Work out the finished part from the listing and answer in its coordinate system (mm). A direction names the side the tool comes from. Round coordinates to 2 decimals unless told otherwise and drop trailing zeros. Write each loop counter-clockwise with the first axis right and the second up, starting at its lowest first coordinate (ties: lowest second). Pieces come first, ordered by that corner, then holes. Notation, with made-up numbers: M 45.5,45 L 103.5,45 A14 cw 103.5,58 Z; hole C -32.5,72.5 d2. An arc over 180 degrees is marked long. One line per item, written item: value. Start each with the question number.
Q1. Find section B-B (x = -47.5). Write down the section's boundary in (y, z).
Q2. Find section A-A (y = -36). Write down the section's boundary in (x, z), and give its area (3 significant figures).
Q3. Given pin 1 Ø9.5 at (x, z) = (-54, 14.5) entering from +Y; pin 2 Ø6 at (y, z) = (-36.5, 6) entering from -X; pin 3 Ø5 at (x, z) = (59.5, 10.5) entering from +Y; pin 4 Ø4 at (x, y) = (-71, -22.5) entering from -Z, each flat-ended and moving along its own axis, determine where each tip first touches the part or whether it passes through.
Q4. Find section C-C (y = -12). Write down the section's boundary in (x, z).
Q5. A tool of negligible diameter and unlimited length cuts with its end or side. For faces 4 (the cylindrical face through (-20.524, -42.135, 10.367)), 5 (the flat face through (64.972, -31, 10)), 6 (the flat face through (78, 26.791, 12)), from which of +Z, -Z, +X, -X, +Y, -Y can it reach the whole face along a straight path? Write none if from no direction.
Q6. Consider probe 1 along X at (y, z) = (30.7, 10); probe 2 along X at (y, z) = (-19.5, 16.75); probe 3 along X at (y, z) = (-50, 12.75). Determine where each line is inside the solid, lowest interval first.
Q7. The mould has two halves that part along Z. Classify faces 1 (the flat face through (-5, -44, 20)), 2 (the conical face through (79.876, 29.058, 10.66)), 3 (the flat face through (-4, -40.709, 10)): released by +Z, released by -Z, zero draft, split by the parting line, or undercut.
from build123d import *

# Parameters (mm, degrees)
F1_DEPTH             = 20
F4_D                 = 4.2
F4_CSINK_D           = 8.2
F4_CSINK_ANGLE       = 80
F4_ON_F2_D           = 4.2
F4_ON_F2_CSINK_D     = 8.2
F4_ON_F2_CSINK_ANGLE = 80
F5_T1_DEPTH          = 20
F5_T3_DEPTH          = 25
F6_R                 = 5
F7_R                 = 1


# Not quite as in the source:
# - a fillet or chamfer that OpenCascade refuses, or shapes differently, is made with other operations: its cross-section is extruded or revolved along the edge and cut away or added


with BuildPart() as f1:
    # F0 (on Top) → F1 (new body)
    with BuildSketch(Plane.XY):
        with BuildLine():
            Line((-74.0278660059, -17.2093475759), (-70.5278660059, -17.2093475759))
            Line((-70.5278660059, -17.2093475759), (-70.5278660059, -4.2093475759))
            Line((-70.5278660059, -4.2093475759), (-74.0278660059, -4.2093475759))
            Line((-74.0278660059, -4.2093475759), (-74.0278660059, 33.7906524241))
            Line((-74.0278660059, 33.7906524241), (-81.0278660059, 33.7906524241))
            Line((-81.0278660059, 33.7906524241), (-96.0278660059, 33.7906524241))
            Line((-96.0278660059, 33.7906524241), (-96.0278660059, 26.7906524241))
            Line((-96.0278660059, 26.7906524241), (-86.0278660059, 26.7906524241))
            ThreePointArc((-86.0278660059, 26.7906524241), (-82.4923321, 25.32618633), (-81.0278660059, 21.7906524241))
            Line((-81.0278660059, 21.7906524241), (-81.0278660059, -48.7093475759))
            Line((-81.0278660059, -48.7093475759), (-81.0278660059, -50.7093475759))
            ThreePointArc((-81.0278660059, -50.7093475759), (-79.5633999118, -54.2448814818), (-76.0278660059, -55.7093475759))
            Line((-76.0278660059, -55.7093475759), (-48.0278660059, -55.7093475759))
            Line((-48.0278660059, -55.7093475759), (-4.5278660059, -55.7093475759))
            Line((-4.5278660059, -55.7093475759), (38.9721339941, -55.7093475759))
            Line((38.9721339941, -55.7093475759), (66.9721339941, -55.7093475759))
            ThreePointArc((66.9721339941, -55.7093475759), (70.5076679, -54.2448814818), (71.9721339941, -50.7093475759))
            Line((71.9721339941, -50.7093475759), (71.9721339941, -48.7093475759))
            Line((71.9721339941, -48.7093475759), (71.9721339941, 21.7906524241))
            ThreePointArc((71.9721339941, 21.7906524241), (73.4366000882, 25.32618633), (76.9721339941, 26.7906524241))
            Line((76.9721339941, 26.7906524241), (86.9721339941, 26.7906524241))
            Line((86.9721339941, 26.7906524241), (86.9721339941, 33.7906524241))
            Line((86.9721339941, 33.7906524241), (71.9721339941, 33.7906524241))
            Line((71.9721339941, 33.7906524241), (64.9721339941, 33.7906524241))
            Line((64.9721339941, 33.7906524241), (64.9721339941, -4.2093475759))
            Line((64.9721339941, -4.2093475759), (61.4721339941, -4.2093475759))
            Line((61.4721339941, -4.2093475759), (61.4721339941, -17.2093475759))
            Line((61.4721339941, -17.2093475759), (64.9721339941, -17.2093475759))
            Line((64.9721339941, -17.2093475759), (64.9721339941, -48.7093475759))
            Line((64.9721339941, -48.7093475759), (12.9721339941, -48.7093475759))
            Line((12.9721339941, -48.7093475759), (12.9721339941, -45.7093475759))
            ThreePointArc((12.9721339941, -45.7093475759), (11.5076679, -42.17381367), (7.9721339941, -40.7093475759))
            Line((7.9721339941, -40.7093475759), (-4.5278660059, -40.7093475759))
            Line((-4.5278660059, -40.7093475759), (-17.0278660059, -40.7093475759))
            ThreePointArc((-17.0278660059, -40.7093475759), (-20.5633999118, -42.17381367), (-22.0278660059, -45.7093475759))
            Line((-22.0278660059, -45.7093475759), (-22.0278660059, -48.7093475759))
            Line((-22.0278660059, -48.7093475759), (-74.0278660059, -48.7093475759))
            Line((-74.0278660059, -48.7093475759), (-74.0278660059, -17.2093475759))
        make_face()
    extrude(amount=F1_DEPTH)

    # F4 (through all)
    with Locations(Plane.XZ.offset(-26.7906524241)):
        with Locations((81.9721339941, 10)):
            CounterSinkHole(F4_D / 2, F4_CSINK_D / 2, counter_sink_angle=F4_CSINK_ANGLE)

    # F4 on F2 (through all)
    with Locations(Plane.XZ.offset(-26.7906524241)):
        with Locations((-91.0278660059, 10)):
            CounterSinkHole(F4_ON_F2_D / 2, F4_ON_F2_CSINK_D / 2, counter_sink_angle=F4_ON_F2_CSINK_ANGLE)

    # F5: fillet of radius 1 on 14 edges, made by hand

    # F5_s2 → F5_t1 (join)
    with BuildSketch(Plane.XY):
        with BuildLine():
            ThreePointArc((-73.0278660059, -4.2093475759), (-73.7349727871, -3.9164543571), (-74.0278660059, -3.2093475759))
            Line((-74.0278660059, -3.2093475759), (-74.0278660059, -4.2093475759))
            Line((-74.0278660059, -4.2093475759), (-73.0278660059, -4.2093475759))
        make_face()
        with BuildLine():
            ThreePointArc((-74.0278660059, -18.2093475759), (-73.7349727871, -17.5022407947), (-73.0278660059, -17.2093475759))
            Line((-73.0278660059, -17.2093475759), (-74.0278660059, -17.2093475759))
            Line((-74.0278660059, -17.2093475759), (-74.0278660059, -18.2093475759))
        make_face()
        with BuildLine():
            ThreePointArc((64.9721339941, -18.2093475759), (64.6792407753, -17.5022407947), (63.9721339941, -17.2093475759))
            Line((63.9721339941, -17.2093475759), (64.9721339941, -17.2093475759))
            Line((64.9721339941, -17.2093475759), (64.9721339941, -18.2093475759))
        make_face()
        with BuildLine():
            ThreePointArc((64.9721339941, -3.2093475759), (64.6792407753, -3.9164543571), (63.9721339941, -4.2093475759))
            Line((63.9721339941, -4.2093475759), (64.9721339941, -4.2093475759))
            Line((64.9721339941, -4.2093475759), (64.9721339941, -3.2093475759))
        make_face()
    extrude(amount=F5_T1_DEPTH)

    # F5_s4 → F5_t3 (cut)
    with BuildSketch(Plane.XY.offset(-2.5)):
        with BuildLine():
            ThreePointArc((65.9721339941, 33.7906524241), (65.2650272129, 33.4977592053), (64.9721339941, 32.7906524241))
            Line((64.9721339941, 32.7906524241), (64.9721339941, 33.7906524241))
            Line((64.9721339941, 33.7906524241), (65.9721339941, 33.7906524241))
        make_face()
        with BuildLine():
            ThreePointArc((62.4721339941, -4.2093475759), (61.7650272129, -4.5022407947), (61.4721339941, -5.2093475759))
            Line((61.4721339941, -5.2093475759), (61.4721339941, -4.2093475759))
            Line((61.4721339941, -4.2093475759), (62.4721339941, -4.2093475759))
        make_face()
        with BuildLine():
            ThreePointArc((61.4721339941, -16.2093475759), (61.7650272129, -16.9164543571), (62.4721339941, -17.2093475759))
            Line((62.4721339941, -17.2093475759), (61.4721339941, -17.2093475759))
            Line((61.4721339941, -17.2093475759), (61.4721339941, -16.2093475759))
        make_face()
        with BuildLine():
            ThreePointArc((-71.5278660059, -17.2093475759), (-70.8207592247, -16.9164543571), (-70.5278660059, -16.2093475759))
            Line((-70.5278660059, -16.2093475759), (-70.5278660059, -17.2093475759))
            Line((-70.5278660059, -17.2093475759), (-71.5278660059, -17.2093475759))
        make_face()
        with BuildLine():
            ThreePointArc((-74.0278660059, 32.7906524241), (-74.3207592247, 33.4977592053), (-75.0278660059, 33.7906524241))
            Line((-75.0278660059, 33.7906524241), (-74.0278660059, 33.7906524241))
            Line((-74.0278660059, 33.7906524241), (-74.0278660059, 32.7906524241))
        make_face()
        with BuildLine():
            ThreePointArc((85.9721339941, 26.7906524241), (86.6792407753, 27.0835456429), (86.9721339941, 27.7906524241))
            Line((86.9721339941, 27.7906524241), (86.9721339941, 26.7906524241))
            Line((86.9721339941, 26.7906524241), (85.9721339941, 26.7906524241))
        make_face()
        with BuildLine():
            ThreePointArc((86.9721339941, 32.7906524241), (86.6792407753, 33.4977592053), (85.9721339941, 33.7906524241))
            Line((85.9721339941, 33.7906524241), (86.9721339941, 33.7906524241))
            Line((86.9721339941, 33.7906524241), (86.9721339941, 32.7906524241))
        make_face()
        with BuildLine():
            ThreePointArc((-70.5278660059, -5.2093475759), (-70.8207592247, -4.5022407947), (-71.5278660059, -4.2093475759))
            Line((-71.5278660059, -4.2093475759), (-70.5278660059, -4.2093475759))
            Line((-70.5278660059, -4.2093475759), (-70.5278660059, -5.2093475759))
        make_face()
        with BuildLine():
            ThreePointArc((-95.0278660059, 33.7906524241), (-95.7349727871, 33.4977592053), (-96.0278660059, 32.7906524241))
            Line((-96.0278660059, 32.7906524241), (-96.0278660059, 33.7906524241))
            Line((-96.0278660059, 33.7906524241), (-95.0278660059, 33.7906524241))
        make_face()
        with BuildLine():
            ThreePointArc((-96.0278660059, 27.7906524241), (-95.7349727871, 27.0835456429), (-95.0278660059, 26.7906524241))
            Line((-95.0278660059, 26.7906524241), (-96.0278660059, 26.7906524241))
            Line((-96.0278660059, 26.7906524241), (-96.0278660059, 27.7906524241))
        make_face()
    extrude(amount=F5_T3_DEPTH, mode=Mode.SUBTRACT)

    # F6
    f6_edges = [f1.edges().sort_by_distance(p)[0] for p in [
        (64.972134, -48.709348, 10),
        (-74.027866, -48.709348, 10),
    ]]
    fillet(f6_edges, radius=F6_R)

    # F7
    f7_edges = [f1.edges().sort_by_distance(p)[0] for p in [
        (-74.027866, -30.959348, 0),
        (-72.5634, -47.244881, 0),
        (-73.734973, -17.502241, 0),
        (-45.527866, -48.709348, 0),
        (-72.277866, -17.209348, 0),
        (-22.027866, -47.209348, 0),
        (-70.820759, -16.916454, 0),
        (-20.5634, -42.173814, 0),
        (-70.527866, -10.709348, 0),
        (-4.527866, -40.709348, 0),
        (-70.820759, -4.502241, 0),
        (11.507668, -42.173814, 0),
        (-72.277866, -4.209348, 0),
        (12.972134, -47.209348, 0),
        (-73.734973, -3.916454, 0),
        (36.472134, -48.709348, 0),
        (-74.027866, 14.790652, 0),
        (63.507668, -47.244881, 0),
        (-74.320759, 33.497759, 0),
        (64.972134, -30.959348, 0),
        (-85.027866, 33.790652, 0),
        (64.679241, -17.502241, 0),
        (-95.734973, 33.497759, 0),
        (63.222134, -17.209348, 0),
        (-96.027866, 30.290652, 0),
        (61.765027, -16.916454, 0),
        (-95.734973, 27.083546, 0),
        (61.472134, -10.709348, 0),
        (-90.527866, 26.790652, 0),
        (61.765027, -4.502241, 0),
        (-82.492332, 25.326186, 0),
        (63.222134, -4.209348, 0),
        (-81.027866, -14.459348, 0),
        (64.679241, -3.916454, 0),
        (-79.5634, -54.244881, 0),
        (64.972134, 14.790652, 0),
        (-4.527866, -55.709348, 0),
        (65.265027, 33.497759, 0),
        (70.507668, -54.244881, 0),
        (75.972134, 33.790652, 0),
        (71.972134, -14.459348, 0),
        (86.679241, 33.497759, 0),
        (73.4366, 25.326186, 0),
        (86.972134, 30.290652, 0),
        (81.472134, 26.790652, 0),
        (86.679241, 27.083546, 0),
    ]]
    fillet(f7_edges, radius=F7_R)


solid = f1.part
The answers:
1. outline: M -55.71,1 A1 ccw -54.71,0 L -49.71,0 A1 ccw -48.71,1 L -48.71,20 L -55.71,20 Z
2. outline: M -81.03,1 A1 ccw -80.03,0 L -75.03,0 A1 ccw -74.03,1 L -74.03,20 L -81.03,20 Z; M 64.97,1 A1 ccw 65.97,0 L 70.97,0 A1 ccw 71.97,1 L 71.97,20 L 64.97,20 Z
2. area: 279 mm2
3. pin 1: y = -48.71
3. pin 2: x = -81.03
3. pin 3: y = -4.33
3. pin 4: through
4. outline: M -81.03,1 A1 ccw -80.03,0 L -71.53,0 A1 ccw -70.53,1 L -70.53,20 L -81.03,20 Z; M 61.47,1 A1 ccw 62.47,0 L 70.97,0 A1 ccw 71.97,1 L 71.97,20 L 61.47,20 Z
5. face 4: +Z, -Z, +Y
5. face 5: +Z, -Z
5. face 6: +Z, -Z, +X, -Y
6. probe 1: -96.03 to -93.13, -88.93 to -74.03, 64.97 to 79.87, 84.07 to 86.97
6. probe 2: -81.03 to -74.03, 64.97 to 71.97
6. probe 3: -81.03 to 71.97
7. face 1: released by +Z
7. face 2: undercut
7. face 3: zero draft
